Work out the finished part from the listing and answer in its coordinate system (mm). A direction names the side the tool comes from. Round coordinates to 2 decimals unless told otherwise and drop trailing zeros. Write each loop counter-clockwise with the first axis right and the second up, starting at its lowest first coordinate (ties: lowest second). Pieces come first, ordered by that corner, then holes. Notation, with made-up numbers: M 16,-23 L 29,-23 A32 cw 29,9 Z; hole C 31,-36 d11. An arc over 180 degrees is marked long. Answer in a Markdown table with one row per item.
Solid Edge part; units mm, degrees
sketch "Sketch1" plane through (0, 0, 0) normal (0, 0, 1) x (1, 0, 0)
  line L0 (27, 25) -> (-27, 25)
  line L1 (-27, 25) -> (-27, 0)
  line L2 (-27, 0) -> (27, 0)
  line L3 (27, 0) -> (27, 25)
  circle A0 centre (14, 19) radius 1.7
  circle A1 centre (-14, 19) radius 1.7
  dimension "D1" = 27
  dimension "D2" = 27
  dimension "D3" = 27
extrude "Protrusion1" add sketch "Sketch1" along normal blind 1.6
sketch "Sketch2" plane through (0, 12.5, 1.6) normal (0, 0, 1) x (1, 0, 0)
  line L0 (-15.75, 1.25) -> (-25.75, 1.25)
  line L1 (-25.75, 1.25) -> (-25.75, -5.25)
  line L2 (-25.75, -5.25) -> (-15.75, -5.25)
  line L3 (-15.75, -5.25) -> (-15.75, 1.25)
  line L4 (-4, 1.25) -> (-14, 1.25)
  line L5 (-14, 1.25) -> (-14, -5.25)
  line L6 (-14, -5.25) -> (-4, -5.25)
  line L7 (-4, -5.25) -> (-4, 1.25)
  line L8 (14, 1.25) -> (4, 1.25)
  line L9 (4, 1.25) -> (4, -5.25)
  line L10 (4, -5.25) -> (14, -5.25)
  line L11 (14, -5.25) -> (14, 1.25)
  line L12 (25.75, 1.25) -> (15.75, 1.25)
  line L13 (15.75, 1.25) -> (15.75, -5.25)
  line L14 (15.75, -5.25) -> (25.75, -5.25)
  line L15 (25.75, -5.25) -> (25.75, 1.25)
  dimension "D1" = 15.75
  dimension "D2" = 25.75
extrude "Buttons" cut sketch "Sketch2" against normal blind 0.3
1. Determine the mould class of faces 3 (the flat face through (0, 0, 1)), 4 (the flat face through (27, 12, 1)), 5 (the flat face through (9, 11, 1.3)) for opening direction Y: released by +Y, released by -Y, zero draft, split by the parting line, or undercut.
Calculated:
| item | result |
|---|---|
| face 3 | released by -Y |
| face 4 | zero draft |
| face 5 | undercut |
2. Consider line 1 along X through (y, z) = (11.75, 1.4); line 2 along Y through (x, z) = (-5, 1.5); line 3 along X through (y, z) = (20.5, 0.45). Determine where each line is inside the solid, lowest interval first. Write a range as from..to.
Calculated:
| item | result |
|---|---|
| line 1 | x = -27..-25.75, -15.75..-14, -4..4, 14..15.75, 25.75..27 |
| line 2 | y = 0..7.25, 13.75..25 |
| line 3 | x = -27..-14.8, -13.2..13.2, 14.8..27 |
3. A tool of negligible diameter and unlimited length cuts with its end or side. For faces 1 (the cylindrical face through (14.914, 17.567, 0.789)), 2 (the flat face through (21, 11, 1.3)), from which of +Z, -Z, +X, -X, +Y, -Y can it reach the whole face along a straight path? Write none if from no direction.
Calculated:
| item | result |
|---|---|
| face 1 | +Z, -Z |
| face 2 | +Z |
4. The part is cut by section A-A (y = 9.25). Determine the outline of the cut face in (x, z), plus the area to 3 significant figures.
Calculated:
| item | result |
|---|---|
| outline | M -27,0 L 27,0 L 27,1.6 L 25.75,1.6 L 25.75,1.3 L 15.75,1.3 L 15.75,1.6 L 14,1.6 L 14,1.3 L 4,1.3 L 4,1.6 L -4,1.6 L -4,1.3 L -14,1.3 L -14,1.6 L -15.75,1.6 L -15.75,1.3 L -25.75,1.3 L -25.75,1.6 L -27,1.6 Z |
| area | 74.4 mm² |
5. The part is cut by section B-B (x = 15). Determine the outline of the cut face in (y, z).
Calculated:
| item | result |
|---|---|
| outline | M 0,0 L 17.63,0 L 17.63,1.6 L 0,1.6 Z; M 20.37,0 L 25,0 L 25,1.6 L 20.37,1.6 Z |
6. The part is cut by section C-C (y = 18). Determine the outline of the cut face in (x, z).
Calculated:
| item | result |
|---|---|
| outline | M -27,0 L -15.37,0 L -15.37,1.6 L -27,1.6 Z; M -12.63,0 L 12.63,0 L 12.63,1.6 L -12.63,1.6 Z; M 15.37,0 L 27,0 L 27,1.6 L 15.37,1.6 Z |
